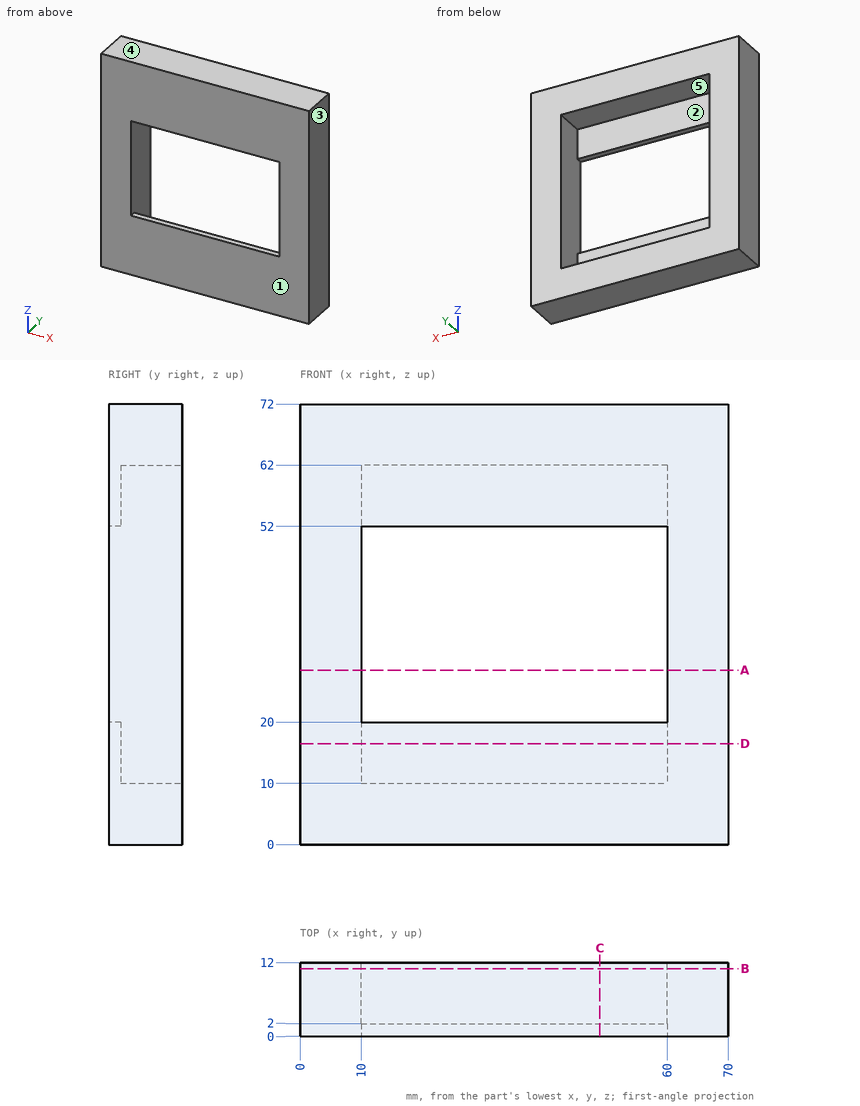
Part print with two shaded views. Sizes in mm from the minimum x, y, z corner. A direction names the side the tool comes from. Round coordinates to 2 decimals unless told otherwise and drop trailing zeros. Order: outer loops, then holes, each group sorted by start corner. A loop starts at its lowest first (then second) coordinate and runs counter-clockwise, first axis right, second up. Notation, with made-up numbers: M 22.25,-22 L 65.25,-22 A35 cw 65.25,11 Z; hole C 74.25,66 d5. An arc over 180 degrees is marked long. Use CSV: the item, a comma, the result in double quotes. Start each with the question number.
(1) Mould opens along X. For the marked faces 3, 4 and 5 say: +X half, -X half, draft (parallel to the pull), parting line (faces both ways), or undercut.
(2) Drill centre lines: probe 1 along X at (y, z) = (11.25, 42.5); probe 2 along Z at (x, y) = (18, 2.5); probe 3 along Y at (x, z) = (55, 55). Where is each one in solid material? Low to high.
(3) Cut at D-D on z = 16.5. List the corners of the cut face in (x, y), then the cut area to 3 significant figures.
(4) Tool access for the marked faces 1 and 2: list every direction of +Z, -Z, +X, -X, +Y, -Y with a clear straight run to the whole face (end or side of a thin tool).
(5) Cut at A-A on z = 28.5. List the corners of the cut face in (x, y).
(6) Cut at C-C on x = 49. List the corners of the cut face in (y, z), then the cut area to 3 significant figures.
(7) Cut at B-B on y = 11. List the corners of the cut face in (x, z), then the cut area to 3 significant figures.
(8) Flat gauge pin, fed straight in: P1, Ø3, axis at x = 23.5, z = 58, coming from the +Y side. Where does the tip first touch, or does it go through?
Findings:
1,face 3,"+X half"
1,face 4,"draft"
1,face 5,"undercut"
2,probe 1,"x = 0 to 10, 60 to 70"
2,probe 2,"z = 0 to 10, 62 to 72"
2,probe 3,"y = 0 to 2"
3,outline,"M 0,0 L 70,0 L 70,12 L 60,12 L 60,2 L 10,2 L 10,12 L 0,12 Z"
3,area,"340 mm^2"
4,face 1,"+Z, -Z, +X, -X, -Y"
4,face 2,"+Y"
5,outline,"M 0,0 L 10,0 L 10,12 L 0,12 Z; M 60,0 L 70,0 L 70,12 L 60,12 Z"
6,outline,"M 0,0 L 12,0 L 12,10 L 2,10 L 2,20 L 0,20 Z; M 0,52 L 2,52 L 2,62 L 12,62 L 12,72 L 0,72 Z"
6,area,"280 mm^2"
7,outline,"M 0,0 L 70,0 L 70,72 L 0,72 Z; hole M 10,10 L 60,10 L 60,62 L 10,62 Z"
7,area,"2,440 mm^2"
8,P1,"stops at y = 2"
